```python
from build123d import *

# Parameters (mm, degrees)
SKETCH1_R                      = 10
BOSS_EXTRUDE1_DEPTH            = 45
CUT_EXTRUDE1_REACH             = 153.52
SKETCH2_W                      = 25
SKETCH2_H                      = 92
CUT_EXTRUDE1_DIRECTION_2_REACH = 153.52
FILLET2_R                      = 10
FILLET3_R                      = 10
CUT_EXTRUDE5_REACH             = 164.244
SKETCH4_W                      = 12
SKETCH4_H                      = 65
CUT_EXTRUDE5_DIRECTION_2_REACH = 164.244
FILLET4_R                      = 25
CHAMFER1_SIZE                  = 5


with BuildPart() as part:
    # Sketch1 → Boss-Extrude1 (new body)
    with BuildSketch(Plane.XY):
        with BuildLine():
            Line((-25, 0), (-25, -11.491470389))
            Line((-25, -11.491470389), (-63.508529611, -50))
            Line((-63.508529611, -50), (-25.980762114, -115))
            ThreePointArc((-25.980762114, -115), (0, -130), (25.980762114, -115))
            Line((25.980762114, -115), (63.508529611, -50))
            Line((63.508529611, -50), (25, -11.491470389))
            Line((25, -11.491470389), (25, 0))
            ThreePointArc((25, 0), (0, 25), (-25, 0))
        make_face()
        Circle(SKETCH1_R, mode=Mode.SUBTRACT)
        with Locations((0, -100)):
            Circle(SKETCH1_R, mode=Mode.SUBTRACT)
    extrude(amount=-BOSS_EXTRUDE1_DEPTH)

    # Sketch2 → Cut-Extrude1 (cut, up to next)
    with BuildSketch(Plane(origin=(0, 0, 0), x_dir=(0, 0, -1), z_dir=(1, 0, 0)), mode=Mode.PRIVATE) as cut_extrude1_sk1:
        with Locations((22.5, -84)):
            Rectangle(SKETCH2_W, SKETCH2_H)
    cut_extrude1_tool1 = extrude(cut_extrude1_sk1.sketch, amount=-CUT_EXTRUDE1_REACH, mode=Mode.PRIVATE) & part.part
    add(cut_extrude1_tool1.solids().sort_by_distance((0, -84, -22.5))[0], mode=Mode.SUBTRACT)

    # Sketch2 → Cut-Extrude1 direction 2 (cut, up to next)
    with BuildSketch(Plane(origin=(0, 0, 0), x_dir=(0, 0, -1), z_dir=(1, 0, 0)), mode=Mode.PRIVATE) as cut_extrude1_direction_2_sk1:
        with Locations((22.5, -84)):
            Rectangle(SKETCH2_W, SKETCH2_H)
    cut_extrude1_direction_2_tool1 = extrude(cut_extrude1_direction_2_sk1.sketch, amount=CUT_EXTRUDE1_DIRECTION_2_REACH, mode=Mode.PRIVATE) & part.part
    add(cut_extrude1_direction_2_tool1.solids().sort_by_distance((0, -84, -22.5))[0], mode=Mode.SUBTRACT)

    # Fillet2
    fillet2_edges = [part.edges().sort_by_distance(p)[0] for p in [
        (25, -11.491470389, -22.5),
        (63.508529611, -50, -40),
        (-63.508529611, -50, -40),
        (-25, -11.491470389, -22.5),
        (-63.508529611, -50, -5),
        (63.508529611, -50, -5),
    ]]
    fillet(fillet2_edges, radius=FILLET2_R)

    # Fillet3
    fillet3_edges = [part.edges().sort_by_distance(p)[0] for p in [
        (0, -38, -10),
        (0, -38, -35),
    ]]
    fillet(fillet3_edges, radius=FILLET3_R)

    # Sketch4 → Cut-Extrude5 (cut, up to next)
    with BuildSketch(Plane(origin=(25, 0, 0), x_dir=(0, 0, -1), z_dir=(1, 0, 0)), mode=Mode.PRIVATE) as cut_extrude5_sk1:
        with Locations((39, -7.5)):
            Rectangle(SKETCH4_W, SKETCH4_H)
    cut_extrude5_tool1 = extrude(cut_extrude5_sk1.sketch, amount=-CUT_EXTRUDE5_REACH, mode=Mode.PRIVATE) & part.part
    # Sketch4 → Cut-Extrude5 (cut, up to next)
    with BuildSketch(Plane(origin=(25, 0, 0), x_dir=(0, 0, -1), z_dir=(1, 0, 0)), mode=Mode.PRIVATE) as cut_extrude5_sk2:
        with Locations((6, -7.5)):
            Rectangle(SKETCH4_W, SKETCH4_H)
    cut_extrude5_tool2 = extrude(cut_extrude5_sk2.sketch, amount=-CUT_EXTRUDE5_REACH, mode=Mode.PRIVATE) & part.part
    add(cut_extrude5_tool1.solids().sort_by_distance((25, -7.5, -39))[0], mode=Mode.SUBTRACT)
    add(cut_extrude5_tool2.solids().sort_by_distance((25, -7.5, -6))[0], mode=Mode.SUBTRACT)

    # Sketch4 → Cut-Extrude5 direction 2 (cut, up to next)
    with BuildSketch(Plane(origin=(25, 0, 0), x_dir=(0, 0, -1), z_dir=(1, 0, 0)), mode=Mode.PRIVATE) as cut_extrude5_direction_2_sk1:
        with Locations((39, -7.5)):
            Rectangle(SKETCH4_W, SKETCH4_H)
    cut_extrude5_direction_2_tool1 = extrude(cut_extrude5_direction_2_sk1.sketch, amount=CUT_EXTRUDE5_DIRECTION_2_REACH, mode=Mode.PRIVATE) & part.part
    # Sketch4 → Cut-Extrude5 direction 2 (cut, up to next)
    with BuildSketch(Plane(origin=(25, 0, 0), x_dir=(0, 0, -1), z_dir=(1, 0, 0)), mode=Mode.PRIVATE) as cut_extrude5_direction_2_sk2:
        with Locations((6, -7.5)):
            Rectangle(SKETCH4_W, SKETCH4_H)
    cut_extrude5_direction_2_tool2 = extrude(cut_extrude5_direction_2_sk2.sketch, amount=CUT_EXTRUDE5_DIRECTION_2_REACH, mode=Mode.PRIVATE) & part.part
    add(cut_extrude5_direction_2_tool1.solids().sort_by_distance((25, -7.5, -39))[0], mode=Mode.SUBTRACT)
    add(cut_extrude5_direction_2_tool2.solids().sort_by_distance((25, -7.5, -6))[0], mode=Mode.SUBTRACT)

    # Fillet4
    # the kernel refuses this fillet: 25 mm, written as the material it adds along each edge
    with BuildSketch(Plane(origin=(-106.893920871, -40, -33), x_dir=(0, 1, 0), z_dir=(1, 0, 0))) as fillet4_piece_1_section:
        with BuildLine():
            CenterArc((21.354156504, -25), FILLET4_R, 90, 58.667748502)
            Line((0, -12), (-0.42708313, -11.74))
            ThreePointArc((-0.42708313, -11.74), (-0.5, -6), (-0.5, 0))
            Line((-0.5, 0), (0, 0.5))
            Line((0, 0.5), (21.354156504, 0.5))
            Line((21.354156504, 0.5), (21.354156504, 0))
        make_face()
    fillet4_piece_1 = extrude(amount=213.787841742, mode=Mode.PRIVATE)
    fillet4_piece_1 = split(fillet4_piece_1, bisect_by=Plane(origin=(-24.314247143, -10.805717532, -36.275046533), z_dir=(0.7071067811865465, -0.7071067811865487, 0)), keep=Keep.TOP, mode=Mode.PRIVATE)
    fillet4_piece_1 = split(fillet4_piece_1, bisect_by=Plane(origin=(24.314247143, -10.805717532, -36.275046533), z_dir=(-0.7071067811865465, -0.7071067811865487, 0)), keep=Keep.TOP, mode=Mode.PRIVATE)
    add(fillet4_piece_1)
    with BuildSketch(Plane(origin=(-106.893920871, -40, -12), x_dir=(0, 0, 1), z_dir=(1, 0, 0))) as fillet4_piece_2_section:
        with BuildLine():
            CenterArc((25, -21.354156504), FILLET4_R, 121.332251498, 58.667748502)
            Line((0, -21.354156504), (-0.5, -21.354156504))
            Line((-0.5, -21.354156504), (-0.5, 0))
            Line((-0.5, 0), (0, 0.5))
            ThreePointArc((0, 0.5), (6, 0.5), (11.74, 0.42708313))
            Line((11.74, 0.42708313), (12, 0))
        make_face()
    fillet4_piece_2 = extrude(amount=213.787841742, mode=Mode.PRIVATE)
    fillet4_piece_2 = split(fillet4_piece_2, bisect_by=Plane(origin=(-24.314247143, -10.805717532, -8.724953467), z_dir=(0.7071067811865465, -0.7071067811865487, 0)), keep=Keep.TOP, mode=Mode.PRIVATE)
    fillet4_piece_2 = split(fillet4_piece_2, bisect_by=Plane(origin=(24.314247143, -10.805717532, -8.724953467), z_dir=(-0.7071067811865465, -0.7071067811865487, 0)), keep=Keep.TOP, mode=Mode.PRIVATE)
    add(fillet4_piece_2)

    # Chamfer1
    chamfer1_edges = [part.edges().sort_by_distance(p)[0] for p in [
        (-10, 0, -12),
        (-10, 0, -33),
        (-10, -100, -45),
        (-10, -100, 0),
    ]]
    chamfer(chamfer1_edges, length=CHAMFER1_SIZE)


solid = part.part
```
Input: part model. Units: mm. Frame: model coordinates. A direction names the side the tool comes from. Give positions to 0.01 mm unless a question says otherwise; leave off trailing zeros. Order: outer loops, then holes, each group sorted by start corner. A loop starts at its lowest first (then second) coordinate and runs counter-clockwise, first axis right, second up. Notation, with made-up numbers: M 17,22.5 L 61,22.5 A9 ccw 61,36.5 Z; hole C 52.5,55 d2. An arc over 180 degrees is marked long. One line per question, with ' | ' between items. Start each with the question number.
1. Pull-direction query (Y, two-part tool) for faces 1 (the face through (-1, -74, 0)), 2 (the face through (60.938, -50.431, -39.772)), 3 (the face through (4.614, -108.872, -7.465)); classes: released by +Y, released by -Y, zero draft, split by the parting line, or undercut.
2. Section query C-C (z = -15). Return the cut outline in (x, y), and give its area (3 significant figures).
3. Material intervals for probe 1 along Z at (x, y) = (-20.5, -79.5); probe 2 along Y at (x, z) = (0, -8.35); probe 3 along Y at (x, z) = (-7, -6), sorted ascending. Write a range as [from, to].
4. Access query for faces 4 (the face through (1, -38, -22)), 5 (the face through (25, -4, -22)), 6 (the face through (-25, -4, -22)). Directions: +Z, -Z, +X, -X, +Y, -Y. A direction counts if a zero-diameter tool reaches every point of the face in a straight line with its end or side. Return the directions, or none.
5. Section query D-D (x = -45.5). Return the cut outline in (y, z), and give its area (3 significant figures).
6. Section query B-B (y = -100). Return the cut outline in (x, z).
7. First-contact query: pin 1 Ø8 at (y, z) = (-20, -32) entering from +X; pin 2 Ø1 at (x, z) = (-47, -6) entering from +Y; pin 3 Ø12 at (x, y) = (0, -100) entering from -Z; pin 4 Ø1 at (y, z) = (-45, -5) entering from +X. Flat tips, straight axial feed; report the tip coordinate or a pass-through.
8. Section query A-A (x = 0). Count the separate pieces of the cut face and the enclosed holes in it, and give its area (3 significant figures).
Here are the results:
1) face 1: zero draft | face 2: split by the parting line | face 3: undercut
2) outline: M -52.85,-39.34 L 52.85,-39.34 L 27.93,-14.42 A10 cw 25,-7.35 L 25,0 A25 ccw -25,0 L -25,-7.35 A10 cw -27.93,-14.42 Z; hole C 0,0 d24 | area: 3,280 mm²
3) probe 1: [-45, -35], [-10, 0] | probe 2: [-130, -110], [-90, -31.65] | probe 3: [-129.17, -107.14], [-92.86, -34.89]
4) face 4: +X, -X, -Y | face 5: +Z, -Z, +X, +Y | face 6: +Z, -Z, -X, +Y
5) outline: M -81.19,-45 L -40,-45 A25 cw -31.99,-36.86 L -31.99,-8.14 A25 cw -40,0 L -81.19,0 L -81.19,-10 L -48,-10 A10 cw -38,-20 L -38,-25 A10 cw -48,-35 L -81.19,-35 Z | area: 1,100 mm²
6) outline: M -34.64,-45 L -15,-45 L -10,-40 L -10,-35 L -34.64,-35 Z; M -34.64,-10 L -10,-10 L -10,-5 L -15,0 L -34.64,0 Z; M 10,-40 L 15,-45 L 34.64,-45 L 34.64,-35 L 10,-35 Z; M 10,-10 L 34.64,-10 L 34.64,0 L 15,0 L 10,-5 Z
7) pin 1: x = 37.51 | pin 2: y = -34.29 | pin 3: through | pin 4: x = 58.9
8) separate pieces: 4 | enclosed holes: 0 | area: 2,390 mm²
